Build history of the part. All positions in model axes, mm. A direction names the side the tool comes from. Coordinates: 2 decimals unless noted, no trailing zeros. Write each loop counter-clockwise with the first axis right and the second up, starting at its lowest first coordinate (ties: lowest second). Pieces come first, ordered by that corner, then holes.
```python
from build123d import *

# Parameters (mm, degrees)
F0_W      = 104.648
F0_H      = 38.1
F1_DEPTH  = 58.42
F2_W      = 80.772
F2_H      = 18.796
F3_DEPTH  = 58.42
F5_DEPTH  = 19.304
F6_W      = 9.166194
F6_H      = 38.1
F6_W_2    = 10.16
F7_DEPTH  = 6.604
F9_DEPTH  = 23.876
F11_DEPTH = 23.876


with BuildPart() as f1:
    # F0 (on Front) → F1 (new body)
    with BuildSketch(Plane.XZ):
        with Locations((52.324, 19.05)):
            Rectangle(F0_W, F0_H)
    extrude(amount=F1_DEPTH)

    # F2 (on face) → F3 (cut)
    with BuildSketch(Plane.XZ.offset(58.42)):
        with Locations((64.262, 28.702)):
            Rectangle(F2_W, F2_H)
    extrude(amount=-F3_DEPTH, mode=Mode.SUBTRACT)

    # F4 (on face) → F5 (cut)
    with BuildSketch(Plane.XY.offset(19.304)):
        Polygon((104.648, 0), (56.388, 0), (104.648, -7.62), align=None)
        Polygon((76.2, -39.116), (104.648, -39.116), (104.648, -19.304), (76.2, -19.304), (76.2, -29.21), align=None)
        with BuildLine():
            ThreePointArc((76.2, -19.304), (66.294, -29.21), (76.2, -39.116))
            Line((76.2, -39.116), (76.2, -29.21))
            Line((76.2, -29.21), (76.2, -19.304))
        make_face()
        Polygon((56.388, -58.42), (104.648, -58.42), (104.648, -50.8), align=None)
    extrude(amount=-F5_DEPTH, mode=Mode.SUBTRACT)

    # F6 (on face) → F7 (cut)
    with BuildSketch(Plane(origin=(0, 0, 0), x_dir=(0, -1, 0), z_dir=(-1, 0, 0))):
        with Locations((4.583097, 19.05)):
            Rectangle(F6_W, F6_H)
        with Locations((53.34, 19.05)):
            Rectangle(F6_W_2, F6_H)
    extrude(amount=-F7_DEPTH, mode=Mode.SUBTRACT)

    # F8 (on face) → F9 (cut)
    with BuildSketch(Plane.YZ.offset(23.876)):
        Polygon((-19.3574, 38.1), (0, 26.924), (0, 38.1), align=None)
    extrude(amount=-F9_DEPTH, mode=Mode.SUBTRACT)

    # F10 (on face) → F11 (cut)
    with BuildSketch(Plane.YZ.offset(23.876)):
        Polygon((-58.42, 38.1), (-58.42, 26.924), (-39.0626, 38.1), align=None)
    extrude(amount=-F11_DEPTH, mode=Mode.SUBTRACT)


solid = f1.part
```
1. 3-axis set-ups, long thin cutter, end or side, ignore diameter. For faces 1 (the face through (91, -19.304, 10)), 2 (the face through (6.604, -53, 17)), 3 (the face through (55, -30, 19.304)), 4 (the face through (3, -9.166, 16)), 5 (the face through (104.648, -45, 10)): which of +Z, -Z, +X, -X, +Y, -Y reach the whole face in a straight line?
Computed values:
face 1: +Z, -Z, +X
face 2: +Z, -Z, -X, -Y
face 3: +Z, +X, +Y, -Y
face 4: +Z, -Z, -X, +Y
face 5: +Z, -Z, +X, +Y, -Y
2. Probe line 1 along Z through (x, y) = (45, -36.5); line 2 along X through (y, z) = (-22, 35); line 3 along Y through (x, z) = (99, 17). List the from-to ranges inside material, lowest first.
Computed values:
line 1: z = 0 to 19.3
line 2: x = 0 to 23.88
line 3: y = -51.69 to -39.12, -19.3 to -6.73
3. Flat gauge pins, fed straight in: pin 1 (3 mm diameter, centred on x = 72.5, z = 8, fed in from -Y); pin 2 (5 mm diameter, centred on x = 30, y = -30.5, fed in from +Z); pin 3 (4.5 mm diameter, centred on y = -6, z = 14.5, fed in from -X). Where does each tip first touch, or does it go through?
Computed values:
pin 1: stops at y = -56.11
pin 2: stops at z = 19.3
pin 3: stops at x = 6.6
4. Saw through at D-D on x = 38.5. List the corners of the cut face in (y, z), plus the area to 3 significant figures.
Computed values:
outline: (-58.42, 0) - (0, 0) - (0, 19.3) - (-58.42, 19.3) - close
area: 1,130 mm2
5. Saw through at C-C on y = -29.21. List the corners of the cut face in (x, z).
Computed values:
outline: (0, 0) - (66.29, 0) - (66.29, 19.3) - (23.88, 19.3) - (23.88, 38.1) - (0, 38.1) - close
6. Saw through at A-A on x = 79.5. List the corners of the cut face in (y, z), plus the area to 3 significant figures.
Computed values:
outline: (-54.77, 0) - (-39.12, 0) - (-39.12, 19.3) - (-54.77, 19.3) - close; (-19.3, 0) - (-3.65, 0) - (-3.65, 19.3) - (-19.3, 19.3) - close
area: 604 mm2
7. Mould opens along Y. For faces 6 (the face through (6.604, -5, 16)), 7 (the face through (66.296, -28.992, 9.787)), 8 (the face through (31, 0, 11)), 9 (the face through (90, -39.116, 10)) say: +Y half, -Y half, draft (parallel to the pull), parting line (faces both ways), or undercut.
Computed values:
face 6: draft
face 7: undercut
face 8: +Y half
face 9: undercut
8. Saw through at B-B on z = 16.5. List the corners of the cut face in (x, y).
Computed values:
outline: (0, -48.26) - (6.6, -48.26) - (6.6, -58.42) - (56.39, -58.42) - (104.65, -50.8) - (104.65, -39.12) - (76.2, -39.12) arc R9.91 cw to (76.2, -19.3) - (104.65, -19.3) - (104.65, -7.62) - (56.39, 0) - (6.6, 0) - (6.6, -9.17) - (0, -9.17) - close
